Autodesk Fusion 360 part; units mm, degrees
sketch "Sketch1" plane through (0, 0, 0) normal (0, 0, 1) x (1, 0, 0)
  line L0 (-16, 26) -> (16, 26) construction
  line L1 (16, 26) -> (16, -26) construction
  line L2 (16, -26) -> (-16, -26) construction
  line L3 (-16, -26) -> (-16, 26) construction
  line L4 (-16, 26) -> (16, -26) construction
  line L5 (16, 26) -> (-16, -26) construction
  line L6 (-7.5, 4.3) -> (7.5, 4.3)
  line L7 (7.5, 4.3) -> (7.5, -4.3)
  line L8 (7.5, -4.3) -> (-7.5, -4.3)
  line L9 (-7.5, -4.3) -> (-7.5, 4.3)
  line L10 (-7.5, 4.3) -> (7.5, -4.3) construction
  line L11 (7.5, 4.3) -> (-7.5, -4.3) construction
  line L12 (-20, 30) -> (20, 30)
  line L13 (20, 30) -> (20, -30)
  line L14 (20, -30) -> (-20, -30)
  line L15 (-20, -30) -> (-20, 30)
  line L16 (-20, 30) -> (20, -30) construction
  line L17 (20, 30) -> (-20, -30) construction
  circle A0 centre (-16, -26) radius 1
  circle A1 centre (16, -26) radius 1
  circle A2 centre (-16, 26) radius 1
  circle A3 centre (16, 26) radius 1
  dimension "d1" = 32
  dimension "d2" = 52
  dimension "d3" = 15
  dimension "d4" = 8.6
  dimension "d5" = 40
  dimension "d6" = 60
  dimension "d7" = 2
  dimension "d8" = 2
  dimension "d9" = 2
  dimension "d10" = 2
extrude "Extrude1" add sketch "Sketch1" along normal blind 3.175
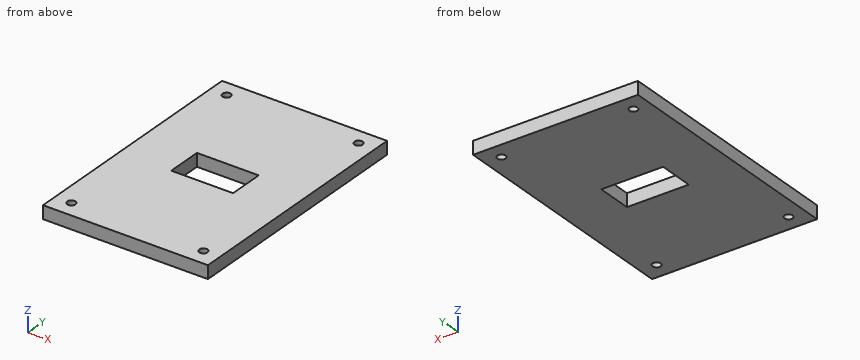
Work out the finished part from the listing and answer in its coordinate system (mm). Round coordinates to 2 decimals unless told otherwise and drop trailing zeros. Write each loop counter-clockwise with the first axis right and the second up, starting at its lowest first coordinate (ties: lowest second). Pieces come first, ordered by that corner, then holes.
1) A cutting plane is placed at B-B on z = 1.7. Determine the outline of the cut face in (x, y).
2) A cutting plane is placed at D-D on x = -6. Determine the outline of the cut face in (y, z) (3 decimals), and give its area (3 significant figures).
3) A cutting plane is placed at A-A on y = -26. Determine the outline of the cut face in (x, z) (3 decimals).
4) Consider probe 1 along Y at (x, z) = (-16, 2.1); probe 2 along Y at (x, z) = (0, 0.7). Determine where each line is inside the solid, lowest interval first.
5) A cutting plane is placed at C-C on x = 16. Determine the outline of the cut face in (y, z) (3 decimals), and give its area (3 significant figures).
Entries:
1. outline: (-20, -30) - (20, -30) - (20, 30) - (-20, 30) - close; hole circle Ø2 at (-16, -26); hole circle Ø2 at (-16, 26); hole (-7.5, -4.3) - (7.5, -4.3) - (7.5, 4.3) - (-7.5, 4.3) - close; hole circle Ø2 at (16, -26); hole circle Ø2 at (16, 26)
2. outline: (-30, 0) - (-4.3, 0) - (-4.3, 3.175) - (-30, 3.175) - close; (4.3, 0) - (30, 0) - (30, 3.175) - (4.3, 3.175) - close
2. area: 163 mm2
3. outline: (-20, 0) - (-17, 0) - (-17, 3.175) - (-20, 3.175) - close; (-15, 0) - (15, 0) - (15, 3.175) - (-15, 3.175) - close; (17, 0) - (20, 0) - (20, 3.175) - (17, 3.175) - close
4. probe 1: y = -30 to -27, -25 to 25, 27 to 30
4. probe 2: y = -30 to -4.3, 4.3 to 30
5. outline: (-30, 0) - (-27, 0) - (-27, 3.175) - (-30, 3.175) - close; (-25, 0) - (25, 0) - (25, 3.175) - (-25, 3.175) - close; (27, 0) - (30, 0) - (30, 3.175) - (27, 3.175) - close
5. area: 178 mm2
